Geometry: final body of the model. Coordinates: model frame, mm. Face numbers are marked on the shaded views. A direction names the side the tool comes from. Coordinates: 2 decimals unless noted, no trailing zeros. Loops run counter-clockwise (first coordinate to the right, second up) from the corner with the lowest first, then second, coordinate; pieces in that order, holes last. Notation, with made-up numbers: (-11.75, 15) -> (10.25, 15) arc R18 ccw to (10.25, 39) -> close; hole circle Ø6 at (-13.75, 28.5). An arc over 180 degrees is marked (long way). One line per item, written item: value. Start each with the question number.
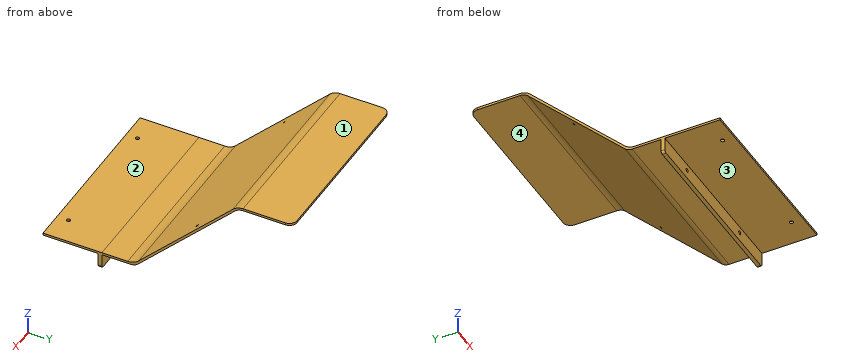
from build123d import *

# Parameters (mm, degrees)
SKETCH1_W           = 250
SKETCH1_H           = 72
BOSS_EXTRUDE1_DEPTH = 3
SKETCH2_W           = 239.6
SKETCH2_H           = 23
BOSS_EXTRUDE2_DEPTH = 5
SKETCH3_R           = 2.5
CUT_EXTRUDE1_DEPTH  = 5
FILLET1_R           = 3
SKETCH4_R           = 2.5
CUT_EXTRUDE2_DEPTH  = 5
SKETCH6_W           = 5.2
SKETCH6_H           = 72
CUT_EXTRUDE3_DEPTH  = 5
BOSS_EXTRUDE3_DEPTH = 239.6
SKETCH8_W           = 239.6
SKETCH8_H           = 3
BOSS_EXTRUDE4_DEPTH = 3
FILLET3_R           = 10
SKETCH10_R          = 1.8
CUT_EXTRUDE5_DEPTH  = 5


with BuildPart() as part:
    # Sketch1 → Boss-Extrude1 (new body)
    with BuildSketch(Plane.XY):
        Rectangle(SKETCH1_W, SKETCH1_H)
    extrude(amount=BOSS_EXTRUDE1_DEPTH)

    # Sketch2 → Boss-Extrude2 (add)
    with BuildSketch(Plane(origin=(0, 36, 0), x_dir=(1, 0, 0), z_dir=(0, 1, 0))):
        with Locations((0, 8.5)):
            Rectangle(SKETCH2_W, SKETCH2_H)
    extrude(amount=BOSS_EXTRUDE2_DEPTH)

    # Sketch3 → Cut-Extrude1 (cut)
    with BuildSketch(Plane(origin=(0, 41, 0), x_dir=(1, 0, 0), z_dir=(0, 1, 0))):
        with Locations(Location((-65, 8.5, 0), (0, 0, 180))):
            Circle(SKETCH3_R)
        with Locations((65, 8.5)):
            Circle(SKETCH3_R)
    extrude(amount=-CUT_EXTRUDE1_DEPTH, mode=Mode.SUBTRACT)

    # Fillet1
    fillet1_edges = [part.edges().sort_by_distance(p)[0] for p in [
        (-119.8, 38.5, -20),
        (119.8, 38.5, -20),
    ]]
    fillet(fillet1_edges, radius=FILLET1_R)

    # Sketch4 → Cut-Extrude2 (cut)
    with BuildSketch(Plane.XY.offset(3)):
        with Locations((-85, -21)):
            Circle(SKETCH4_R)
        with Locations((85, -21)):
            Circle(SKETCH4_R)
    extrude(amount=-CUT_EXTRUDE2_DEPTH, mode=Mode.SUBTRACT)

    # Sketch6 → Cut-Extrude3 (cut)
    with BuildSketch(Plane.XY.offset(3)):
        with Locations((-122.4, 0)):
            Rectangle(SKETCH6_W, SKETCH6_H)
        with Locations((122.4, 0)):
            Rectangle(SKETCH6_W, SKETCH6_H)
    extrude(amount=-CUT_EXTRUDE3_DEPTH, mode=Mode.SUBTRACT)

    # Sketch7 → Boss-Extrude3 (add)
    with BuildSketch(Plane.ZY.offset(119.8)):
        with BuildLine():
            Line((0, 41), (3, 41))
            Line((3, 41), (2.916490723, 74.715728753))
            add(Edge.make_bspline(
                [(2.916490723, 74.715728753), (3.032377234, 82.951998235), (8.774355099, 88.857864376)],
                knots=[0, 0, 0, 1, 1, 1], degree=2))
            Line((8.774355099, 88.857864376), (132.058626347, 212.142135624))
            add(Edge.make_bspline(
                [(132.058626347, 212.142135624), (137.487179548, 217.729604737), (137.916490723, 225.455844123)],
                knots=[0, 0, 0, 1, 1, 1], degree=2))
            Line((137.916490723, 225.455844123), (137.916490723, 287.774355099))
            Line((137.916490723, 287.774355099), (134.916490723, 287.774355099))
            Line((134.916490723, 287.774355099), (134.916490723, 225.455844123))
            ThreePointArc((134.916490723, 225.455844123), (133.774683711, 219.715592637), (130.523092441, 214.849242405))
            Line((130.523092441, 214.849242405), (3.803620061, 88.129770025))
            ThreePointArc((3.803620061, 88.129770025), (0.988528647, 83.916687992), (0, 78.947018888))
            Line((0, 78.947018888), (0, 41))
        make_face()
    extrude(amount=-BOSS_EXTRUDE3_DEPTH)

    # Sketch8 → Boss-Extrude4 (add)
    with BuildSketch(Plane.XY.offset(137.916490723)):
        with Locations((0, 289.274355099)):
            Rectangle(SKETCH8_W, SKETCH8_H)
    extrude(amount=-BOSS_EXTRUDE4_DEPTH)

    # Fillet3
    fillet3_edges = [part.edges().sort_by_distance(p)[0] for p in [
        (-119.8, 290.774355099, 136.416490723),
        (119.8, 290.774355099, 136.416490723),
    ]]
    fillet(fillet3_edges, radius=FILLET3_R)

    # Sketch10 → Cut-Extrude5 (cut)
    with BuildSketch(Plane(origin=(0, 42.163074982, -42.163074982), x_dir=(1, 0, 0), z_dir=(0, 0.7071067811865429, -0.7071067811865522))):
        with Locations(Location((107.5, -168.386692879, 0), (0, 0, 270))):
            Circle(SKETCH10_R)
        with Locations(Location((-107.5, -168.386692879, 0), (0, 0, 270))):
            Circle(SKETCH10_R)
    extrude(amount=-CUT_EXTRUDE5_DEPTH, mode=Mode.SUBTRACT)


solid = part.part
1. Line query: L1, parallel to X at y = 39, z = -8; L2, parallel to Z at x = -101.5, y = 43; L3, parallel to Z at x = 72, y = 264. Output: solid intervals per line, ascending. Write a range as [from, to].
2. Pin query (flat end, axial travel): pin 1 Ø8 at (x, z) = (-65, -8.5) entering from -Y; pin 2 Ø8 at (x, y) = (56.5, 194) entering from -Z; pin 3 Ø1.5 at (x, z) = (30, 102.5) entering from +Y. Return the tip coordinate at first contact, or that it passes through.
3. Section A-A on y = 13.5. Return the cut outline in (x, z), plus the area to 3 significant figures.
4. Set-up query: the marked faces 1, 2, 3 and 4. Return all of +Z, -Z, +X, -X, +Y, -Y with unobstructed straight access to the full face (end or side cutting, diameter ignored); none if empty.
5. Section B-B on z = 91.5. Return the cut outline in (x, y), plus the area to 3 significant figures.
Checks:
1. L1: [-119.8, -67.45], [-62.55, 62.55], [67.45, 119.8]
1. L2: [0, 3]
1. L3: [134.92, 137.92]
2. pin 1: y = 36
2. pin 2: z = 105.67
2. pin 3: y = 187.58
3. outline: (-119.8, 0) -> (119.8, 0) -> (119.8, 3) -> (-119.8, 3) -> close
3. area: 719 mm²
4. face 1: +Z, +X, -X, +Y, -Y
4. face 2: +Z, +X, -X, -Y
4. face 3: -Z, +X, -X, -Y
4. face 4: -Z, +X, -X, +Y
5. outline: (-119.8, 171.58) -> (119.8, 171.58) -> (119.8, 175.83) -> (-119.8, 175.83) -> close
5. area: 1,020 mm²
